Print and shaded views of the part. All mm, measured from the part's lowest x, y and z. A direction names the side the tool comes from. Give positions to 0.01 mm unless a question says otherwise; leave off trailing zeros. Loops run counter-clockwise (first coordinate to the right, second up) from the corner with the lowest first, then second, coordinate; pieces in that order, holes last. Notation, with made-up numbers: M 77.5,12.25 L 110.5,12.25 A18 cw 110.5,45.25 Z; hole C -29.75,4.25 d10. An arc over 180 degrees is marked long. Put each result on its own line as item: value. Start each with the question number.
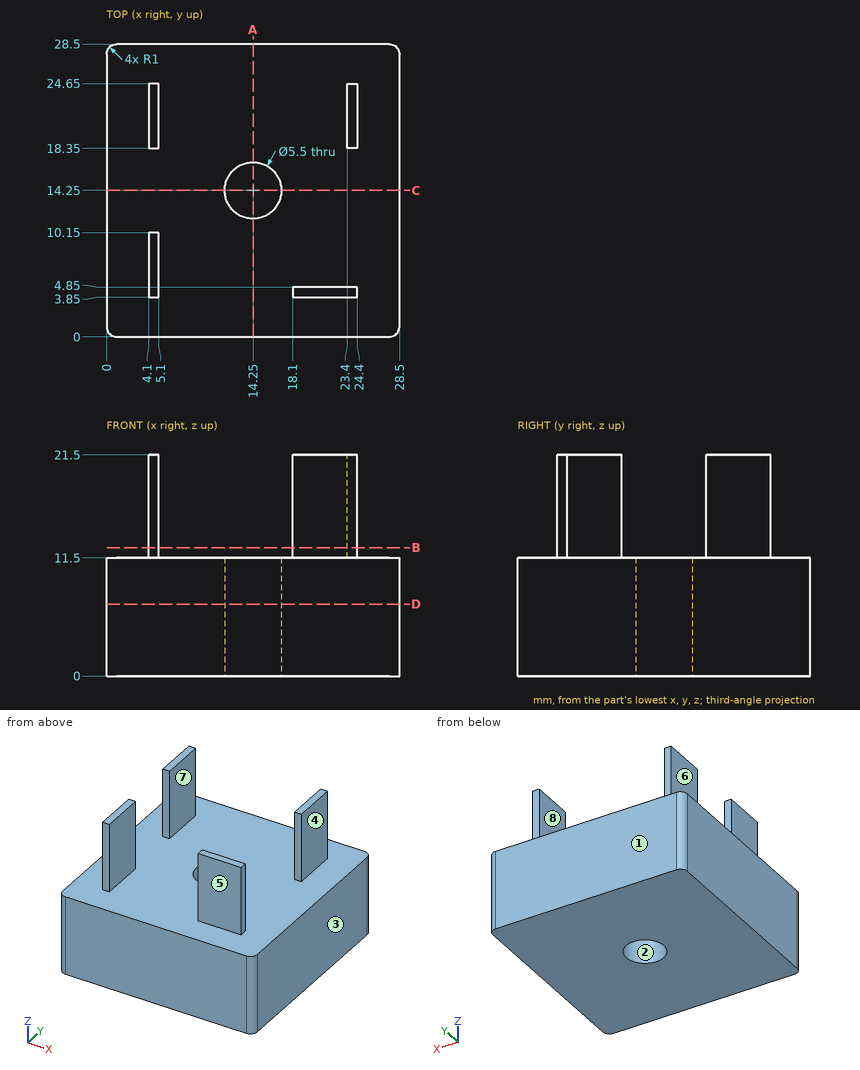
1) Band-saw the part on D-D on z = 7. Give the cut face in (x, y).
2) Band-saw the part on B-B on z = 12.5. Give the cut face in (x, y), then the cut area to 3 significant figures.
3) Which spindle directions (+Z, -Z, +X, -X, +Y, -Y) get a long thin tool onto all of the face, cutting with end or side? Do the marked faces 4, 5, 6, 7 and 8. Say none if no direction does.
4) Band-saw the part on A-A on x = 14.25. Give the cut face in (y, z).
5) Pin check, flat tips, straight feed: pin 1 Ø1.5 at (y, z) = (10, 8.5) entering from -X; pin 2 Ø0.5 at (x, z) = (5, 19) entering from +Y; pin 3 Ø2 at (y, z) = (8.5, 19.5) entering from -X; pin 4 Ø6 at (x, z) = (18, 17.5) entering from -Y. Stop position of each tip, or through.
6) Wall check: L1, parallel to X at y = 14.25, z = 5.75; L2, parallel to Z at x = 22.25, y = 12.75. Give the ranges that are in metal, low to high.
7) Mould opens along X. For the marked faces 1, 2 and 3 say: +X half, -X half, draft (parallel to the pull), parting line (faces both ways), or undercut.
Evaluation:
1. outline: M 0,1 A1 ccw 1,0 L 27.5,0 A1 ccw 28.5,1 L 28.5,27.5 A1 ccw 27.5,28.5 L 1,28.5 A1 ccw 0,27.5 Z; hole C 14.25,14.25 d5.5
2. outline: M 4.1,3.85 L 5.1,3.85 L 5.1,10.15 L 4.1,10.15 Z; M 4.1,18.35 L 5.1,18.35 L 5.1,24.65 L 4.1,24.65 Z; M 18.1,3.85 L 24.4,3.85 L 24.4,4.85 L 18.1,4.85 Z; M 23.4,18.35 L 24.4,18.35 L 24.4,24.65 L 23.4,24.65 Z
2. area: 25.2 mm2
3. face 4: +Z, +X, +Y, -Y
3. face 5: +Z, +X, -X, -Y
3. face 6: +Z, -X, +Y, -Y
3. face 7: +Z, +Y, -Y
3. face 8: +Z, +Y
4. outline: M 0,0 L 11.5,0 L 11.5,11.5 L 0,11.5 Z; M 17,0 L 28.5,0 L 28.5,11.5 L 17,11.5 Z
5. pin 1: x = 0
5. pin 2: y = 24.65
5. pin 3: x = 4.1
5. pin 4: y = 3.85
6. L1: 0 to 11.5, 17 to 28.5
6. L2: 0 to 11.5
7. face 1: draft
7. face 2: undercut
7. face 3: +X half
